Geometry: see drawing. Coordinates: mm, zero at the bounding-box minimum. A direction names the side the tool comes from. Round coordinates to 2 decimals unless told otherwise and drop trailing zeros. Order: outer loops, then holes, each group sorted by start corner. A loop starts at its lowest first (then second) coordinate and runs counter-clockwise, first axis right, second up. Notation, with made-up numbers: (-5.75, 23.25) -> (48.25, 23.25) arc R28 ccw to (48.25, 43.25) -> close; hole circle Ø5 at (34, 52). An arc over 180 degrees is marked (long way). One line per item, written item: value. Start each with the question number.
1) Section A-A (y = 26.5). Return the cut outline in (x, z).
2) Reachability of the marked faces 1, 2, 3, 4 and 5 from +Z, -Z, +X, -X, +Y, -Y: full face, straight path, thin tool, end or side. Return the list, or none.
3) Pin query (flat end, axial travel): P1, Ø8, axis at x = 42, y = 34, coming from the +Z side; P2, Ø1.5, axis at x = 44, z = 4, coming from the -Y side; P3, Ø10, axis at y = 19.5, z = 35, coming from the +X side. Return the tip coordinate at first contact, or that it passes through.
4) Section D-D (y = 19). Return the cut outline in (x, z), and give its area (3 significant figures).
5) Section C-C (y = 4). Return the cut outline in (x, z).
6) Mould query, pull axis X, two halves, no side actions, for the marked faces 6, 7 and 8. Classes: pulls with the +X half, pulls with the -X half, needs draft (parallel to the pull), parting line crosses it, or undercut.
7) Section B-B (z = 13). Return the cut outline in (x, y) (3 decimals).
8) Ray query, L1, parallel to X at y = 13.5, z = 24.5; L2, parallel to X at y = 5.5, z = 13.5; L3, parallel to Z at x = 35, y = 20.5. Return the intervals inside material, ascending.
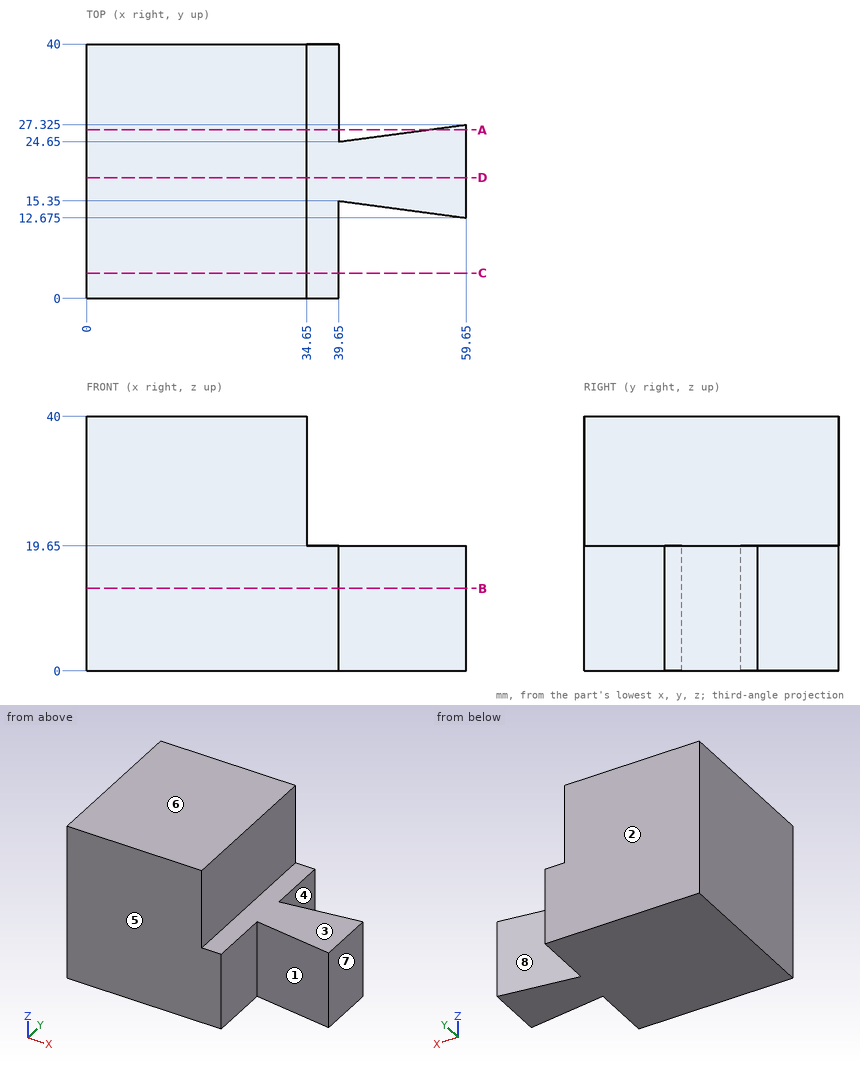
Findings:
1. outline: (0, 0) -> (39.65, 0) -> (39.65, 19.65) -> (34.65, 19.65) -> (34.65, 40) -> (0, 40) -> close; (53.48, 0) -> (59.65, 0) -> (59.65, 19.65) -> (53.48, 19.65) -> close
2. face 1: +Z, -Z, -Y
2. face 2: +Z, -Z, +X, -X, +Y
2. face 3: +Z, +X, +Y, -Y
2. face 4: +Z, -Z, +Y
2. face 5: +Z, -Z, +X, -X, -Y
3. P1: z = 19.65
3. P2: y = 14.67
3. P3: x = 34.65
4. outline: (0, 0) -> (59.65, 0) -> (59.65, 19.65) -> (34.65, 19.65) -> (34.65, 40) -> (0, 40) -> close
4. area: 1,880 mm2
5. outline: (0, 0) -> (39.65, 0) -> (39.65, 19.65) -> (34.65, 19.65) -> (34.65, 40) -> (0, 40) -> close
6. face 6: needs draft
6. face 7: pulls with the +X half
6. face 8: undercut
7. outline: (0, 0) -> (39.65, 0) -> (39.65, 15.35) -> (59.65, 12.675) -> (59.65, 27.325) -> (39.65, 24.65) -> (39.65, 40) -> (0, 40) -> close
8. L1: 0 to 34.65
8. L2: 0 to 39.65
8. L3: 0 to 19.65
